```python
from build123d import *

# Parameters (mm, degrees)
BOSS_EXTRUDE1_DEPTH     = 0.5
SKETCH2_W               = 2
SKETCH2_H               = 10
CUT_EXTRUDE1_DEPTH      = 1.5
CUT_EXTRUDE1_DEPTH_BACK = 1.5
SKETCH3_R               = 0.75
SKETCH3_W               = 8.3
SKETCH3_H               = 3.6
CUT_EXTRUDE2_DEPTH      = 1.5
CUT_EXTRUDE2_DEPTH_BACK = 1.5
SKETCH4_R               = 2.1
BOSS_EXTRUDE2_DEPTH     = 10
SKETCH5_R               = 1.5
BOSS_EXTRUDE3_DEPTH     = 2.5
DOME1_FACE_RADIUS       = 1.5
DOME1_HEIGHT            = 1.5
SKETCH6_W               = 13
SKETCH6_H               = 4
SKETCH6_H_2             = 4.5
BOSS_EXTRUDE4_DEPTH     = 4
BOSS_EXTRUDE5_DEPTH     = 3.5
SKETCH8_R               = 5.65
BOSS_EXTRUDE6_DEPTH     = 3
BOSS_EXTRUDE7_DEPTH     = 3.7
SKETCH11_W              = 8.3
SKETCH11_H              = 2.8
BOSS_EXTRUDE8_DEPTH     = 2.2
CUT_EXTRUDE3_DEPTH      = 3.5
CUT_EXTRUDE4_REACH      = 3
SKETCH15_R              = 0.4


with BuildPart() as part:
    # Sketch1 → Boss-Extrude1 (new body, symmetric)
    with BuildSketch(Plane.XY):
        with BuildLine():
            Line((-19.75, 8.75), (19.75, 8.75))
            ThreePointArc((19.75, 8.75), (28.5, 0), (19.75, -8.75))
            Line((19.75, -8.75), (-19.75, -8.75))
            ThreePointArc((-19.75, -8.75), (-28.5, 0), (-19.75, 8.75))
        make_face()
    extrude(amount=BOSS_EXTRUDE1_DEPTH, both=True)

    # Sketch2 → Cut-Extrude1 (cut, two sides)
    with BuildSketch(Plane.XY) as cut_extrude1_sk:
        with Locations((29.4, 0)):
            Rectangle(SKETCH2_W, SKETCH2_H)
        with Locations((-29.4, 0)):
            Rectangle(SKETCH2_W, SKETCH2_H)
        with BuildLine():
            Line((2.4, 7.55), (-2.4, 7.55))
            ThreePointArc((-2.4, 7.55), (-2.682842712, 7.667157288), (-2.8, 7.95))
            Line((-2.8, 7.95), (-2.8, 9.95))
            Line((-2.8, 9.95), (2.8, 9.95))
            Line((2.8, 9.95), (2.8, 7.95))
            ThreePointArc((2.8, 7.95), (2.682842712, 7.667157288), (2.4, 7.55))
        make_face()
    extrude(amount=CUT_EXTRUDE1_DEPTH, mode=Mode.SUBTRACT)
    extrude(cut_extrude1_sk.sketch, amount=-CUT_EXTRUDE1_DEPTH_BACK, mode=Mode.SUBTRACT)

    # Sketch3 → Cut-Extrude2 (cut, two sides)
    with BuildSketch(Plane.XY) as cut_extrude2_sk:
        with Locations((23.65, 0)):
            Circle(SKETCH3_R)
        with Locations((-18.85, 0)):
            Circle(SKETCH3_R)
        with Locations((17.15, 0)):
            Rectangle(SKETCH3_W, SKETCH3_H)
    extrude(amount=CUT_EXTRUDE2_DEPTH, mode=Mode.SUBTRACT)
    extrude(cut_extrude2_sk.sketch, amount=-CUT_EXTRUDE2_DEPTH_BACK, mode=Mode.SUBTRACT)

    # Sketch4 → Boss-Extrude2 (add)
    with BuildSketch(Plane.XY.offset(0.5)):
        with Locations((-25.8, 0)):
            Circle(SKETCH4_R)
    extrude(amount=BOSS_EXTRUDE2_DEPTH)

    # Sketch5 → Boss-Extrude3 (add)
    with BuildSketch(Plane.XY.offset(10.5)):
        with Locations((-25.8, 0)):
            Circle(SKETCH5_R)
    extrude(amount=BOSS_EXTRUDE3_DEPTH)

    # Dome1: a dome of height H over a round flat face of radius A is a cap of a sphere of radius (A * A + H * H) / (2 * H)
    dome1_r = (DOME1_FACE_RADIUS * DOME1_FACE_RADIUS + DOME1_HEIGHT * DOME1_HEIGHT) / (2 * DOME1_HEIGHT)
    dome1_base = Plane((-25.8, 0, 13), z_dir=(0, 0, 1))
    with Locations(dome1_base.offset(DOME1_HEIGHT - dome1_r)):
        dome1_ball = Sphere(dome1_r, mode=Mode.PRIVATE)
    add(split(dome1_ball, bisect_by=dome1_base, keep=Keep.TOP, mode=Mode.PRIVATE))

    # Sketch6 → Boss-Extrude4 (add)
    with BuildSketch(Plane.XY.offset(0.5)):
        with BuildLine():
            Line((-6.5, -2), (-6.5, 2))
            Line((-6.5, 2), (-9, 2))
            ThreePointArc((-9, 2), (-11, 0), (-9, -2))
            Line((-9, -2), (-6.5, -2))
        make_face()
        Rectangle(SKETCH6_W, SKETCH6_H)
        with BuildLine():
            Line((9, 2), (6.5, 2))
            Line((6.5, 2), (6.5, -2))
            Line((6.5, -2), (9, -2))
            ThreePointArc((9, -2), (11, 0), (9, 2))
        make_face()
        with Locations((0, -4.25)):
            Rectangle(SKETCH6_W, SKETCH6_H_2)
        with Locations((0, 4.25)):
            Rectangle(SKETCH6_W, SKETCH6_H_2)
    extrude(amount=BOSS_EXTRUDE4_DEPTH)

    # Sketch7 → Boss-Extrude5 (add)
    with BuildSketch(Plane.XY.offset(4.5)):
        with BuildLine():
            Line((6.531462317, 1.25), (6.531462317, -1.25))
            ThreePointArc((6.531462317, -1.25), (4.702260095, -4.702260095), (1.25, -6.531462317))
            Line((1.25, -6.531462317), (-1.25, -6.531462317))
            ThreePointArc((-1.25, -6.531462317), (-4.702260095, -4.702260095), (-6.531462317, -1.25))
            Line((-6.531462317, -1.25), (-6.531462317, 1.25))
            ThreePointArc((-6.531462317, 1.25), (-4.702260095, 4.702260095), (-1.25, 6.531462317))
            Line((-1.25, 6.531462317), (1.25, 6.531462317))
            ThreePointArc((1.25, 6.531462317), (4.702260095, 4.702260095), (6.531462317, 1.25))
        make_face()
    extrude(amount=BOSS_EXTRUDE5_DEPTH)

    # Sketch8 → Boss-Extrude6 (add)
    with BuildSketch(Plane.XY.offset(8)):
        Circle(SKETCH8_R)
    extrude(amount=BOSS_EXTRUDE6_DEPTH)

    # Sketch9 → Revolve1 (revolve)
    with BuildSketch(Plane(origin=(0, 0, 0), x_dir=(1, 0, 0), z_dir=(0, 1, 0))):
        with BuildLine():
            Line((0, -11), (7, -11))
            Line((7, -11), (7, -16.9))
            Line((7, -16.9), (5.4, -15.65))
            ThreePointArc((5.4, -15.65), (2.771394054, -16.583422311), (0, -16.9))
            Line((0, -16.9), (0, -11))
        make_face()
    revolve(axis=Axis((0, 0, 0.5), (0, 0, 1)))

    # Sketch10 → Boss-Extrude7 (add)
    with BuildSketch(Plane.XY.offset(0.5)):
        Polygon((10.75, 4.6), (22, 4.6), (22, 6.7), (20.525, 6.7), (20.525, 7.4), (12.225, 7.4), (12.225, 6.7), (10.75, 6.7), align=None)
    extrude(amount=BOSS_EXTRUDE7_DEPTH)

    # Sketch11 → Boss-Extrude8 (add)
    with BuildSketch(Plane.XY.offset(4.2)):
        with Locations((16.375, 6)):
            Rectangle(SKETCH11_W, SKETCH11_H)
    extrude(amount=BOSS_EXTRUDE8_DEPTH)

    # Sketch12 → Cut-Extrude3 (cut)
    with BuildSketch(Plane.XY.offset(6.4)):
        Polygon((20.025, 7.4), (20.025, 6.6), (20.125, 6.6), (20.125, 5.8), (20.025, 5.8), (20.025, 5), (12.725, 5), (12.725, 5.8), (12.625, 5.8), (12.625, 6.6), (12.725, 6.6), (12.725, 7.4), align=None)
    extrude(amount=-CUT_EXTRUDE3_DEPTH, mode=Mode.SUBTRACT)

    # Sketch15 → Cut-Extrude4 (cut, up to next)
    with BuildSketch(Plane.XY.offset(0.5), mode=Mode.PRIVATE) as cut_extrude4_sk1:
        with Locations((11, 8.75)):
            Circle(SKETCH15_R)
    cut_extrude4_tool1 = extrude(cut_extrude4_sk1.sketch, amount=-CUT_EXTRUDE4_REACH, mode=Mode.PRIVATE) & part.part
    add(cut_extrude4_tool1.solids().sort_by_distance((11, 8.75, 0.5))[0], mode=Mode.SUBTRACT)
    # Sketch15 → Cut-Extrude4 (cut, up to next)
    with BuildSketch(Plane.XY.offset(0.5), mode=Mode.PRIVATE) as cut_extrude4_sk2:
        with Locations((-11, 8.75)):
            Circle(SKETCH15_R)
    cut_extrude4_tool2 = extrude(cut_extrude4_sk2.sketch, amount=-CUT_EXTRUDE4_REACH, mode=Mode.PRIVATE) & part.part
    add(cut_extrude4_tool2.solids().sort_by_distance((-11, 8.75, 0.5))[0], mode=Mode.SUBTRACT)
    # Sketch15 → Cut-Extrude4 (cut, up to next)
    with BuildSketch(Plane.XY.offset(0.5), mode=Mode.PRIVATE) as cut_extrude4_sk3:
        with Locations((-11, -8.75)):
            Circle(SKETCH15_R)
    cut_extrude4_tool3 = extrude(cut_extrude4_sk3.sketch, amount=-CUT_EXTRUDE4_REACH, mode=Mode.PRIVATE) & part.part
    add(cut_extrude4_tool3.solids().sort_by_distance((-11, -8.75, 0.5))[0], mode=Mode.SUBTRACT)
    # Sketch15 → Cut-Extrude4 (cut, up to next)
    with BuildSketch(Plane.XY.offset(0.5), mode=Mode.PRIVATE) as cut_extrude4_sk4:
        with Locations((11, -8.75)):
            Circle(SKETCH15_R)
    cut_extrude4_tool4 = extrude(cut_extrude4_sk4.sketch, amount=-CUT_EXTRUDE4_REACH, mode=Mode.PRIVATE) & part.part
    add(cut_extrude4_tool4.solids().sort_by_distance((11, -8.75, 0.5))[0], mode=Mode.SUBTRACT)


solid = part.part
```
Input: part model. Units: mm. Frame: model coordinates. A direction names the side the tool comes from. Round coordinates to 2 decimals unless told otherwise and drop trailing zeros. Loops run counter-clockwise (first coordinate to the right, second up) from the corner with the lowest first, then second, coordinate; pieces in that order, holes last. Notation, with made-up numbers: (21, 84) -> (70, 84) arc R13 cw to (70, 103) -> close; hole circle Ø8 at (82, 36). An arc over 180 degrees is marked (long way). Write each question's results on one line, items separated by ' | '.
1. Section D-D (z = 10). Return loops of the section in (x, y).
Geometry results:
outline: circle Ø4.2 at (-25.8, 0); circle Ø11.3 at (0, 0)
2. First-contact query: P1, Ø1, axis at x = 18, z = 4.5, coming from the +Y side; P2, Ø4.5, axis at y = -4.5, z = 3, coming from the -X side; P3, Ø8, axis at y = 3.5, z = 6, coming from the -X side. Flat tips, straight axial feed; report the tip coordinate or a pass-through.
Geometry results:
P1: y = 5 | P2: x = -6.5 | P3: x = -27.9
3. Section B-B (x = -18.85). Return loops of the section in (y, z), and give its area (3 significant figures).
Geometry results:
outline: (-8.75, -0.5) -> (-0.75, -0.5) -> (-0.75, 0.5) -> (-8.75, 0.5) -> close; (0.75, -0.5) -> (8.75, -0.5) -> (8.75, 0.5) -> (0.75, 0.5) -> close | area: 16.0 mm2
4. Mould query, pull axis Y, two halves, no side actions, for faces 1 (the face through (16, -8.75, 0)), 2 (the face through (13, 0, 0)), 3 (the face through (-4.741, 4.663, 6.226)). Classes: +Y half, -Y half, draft (parallel to the pull), parting line (faces both ways), or undercut.
Geometry results:
face 1: -Y half | face 2: undercut | face 3: +Y half
5. Set-up query: faces 4 (the face through (-6.531, 0, 6)), 5 (the face through (21.3, 0, 0)), 6 (the face through (0, 6.531, 6)), 7 (the face through (6.531, 0, 6)). Return all of +Z, -Z, +X, -X, +Y, -Y with unobstructed straight access to the full face (end or side cutting, diameter ignored); none if empty.
Geometry results:
face 4: +Y, -Y | face 5: +Z, -Z | face 6: -X, +Y | face 7: +X, +Y, -Y
6. Section A-A (z = 1.25). Return loops of the section in (x, y) (3 decimals), and give its area (3 significant figures).
Geometry results:
outline: circle Ø4.2 at (-25.8, 0); (-9, -2) -> (-6.5, -2) -> (-6.5, -6.5) -> (6.5, -6.5) -> (6.5, -2) -> (9, -2) arc R2 ccw to (9, 2) -> (6.5, 2) -> (6.5, 6.5) -> (-6.5, 6.5) -> (-6.5, 2) -> (-9, 2) arc R2 ccw to start; (10.75, 4.6) -> (22, 4.6) -> (22, 6.7) -> (20.525, 6.7) -> (20.525, 7.4) -> (12.225, 7.4) -> (12.225, 6.7) -> (10.75, 6.7) -> close | area: 245 mm2
7. Ray query, line 1 (X direction, y = 0, z = 0.3); line 2 (Y direction, x = -18.85, z = -0.15); line 3 (X direction, y = 7.25, z = 6.25) (3 decimals). Return the intervals inside material, ascending. Write a range as from..to.
Geometry results:
line 1: -28.4..-19.6, -18.1..13, 21.3..22.9, 24.4..28.4 | line 2: -8.75..-0.75, 0.75..8.75 | line 3: 12.225..12.725, 20.025..20.525
